Part print with two shaded views. Sizes in mm from the minimum x, y, z corner. A direction names the side the tool comes from. Coordinates: 2 decimals unless noted, no trailing zeros. Loops run counter-clockwise (first coordinate to the right, second up) from the corner with the lowest first, then second, coordinate; pieces in that order, holes last. Notation, with made-up numbers: (26.25, 20.25) -> (32.25, 20.25) arc R6 cw to (32.25, 27.25) -> close; hole circle Ø9 at (-34, -30.75). An arc over 180 degrees is marked (long way). Return JSON: item names as keys, results as strings. Group by question number.
(1) Saw through at C-C on y = 53.5. Write the cut outline in (x, z).
(2) Mould opens along Y. For the marked faces 3, 4, 5 and 6 say: pulls with the +Y half, pulls with the -Y half, needs draft (parallel to the pull), parting line crosses it, or undercut.
(3) Flat gauge pin, fed straight in: pin 1 Ø11 at (x, y) = (90, 22) entering from +Z. Where does the tip first touch, or does it go through?
(4) Saw through at D-D on z = 6.5. Write the cut outline in (x, y).
(5) Saw through at A-A on x = 39.5. Write the cut outline in (y, z), then the cut area to 3 significant figures.
(6) Probe L1, parallel to Y at x = 106.5, z = 1.55; L2, parallel to X at y = 84, z = 13; L3, parallel to Y at x = 114, z = 11. List the from-to ranges inside material, lowest first.
(7) Tool access for the marked faces 1 and 2: list every direction of +Z, -Z, +X, -X, +Y, -Y with a clear straight run to the whole face (end or side of a thin tool).
(8) Saw through at B-B on y = 87.5. Write the cut outline in (x, z), then the cut area to 3 significant figures.
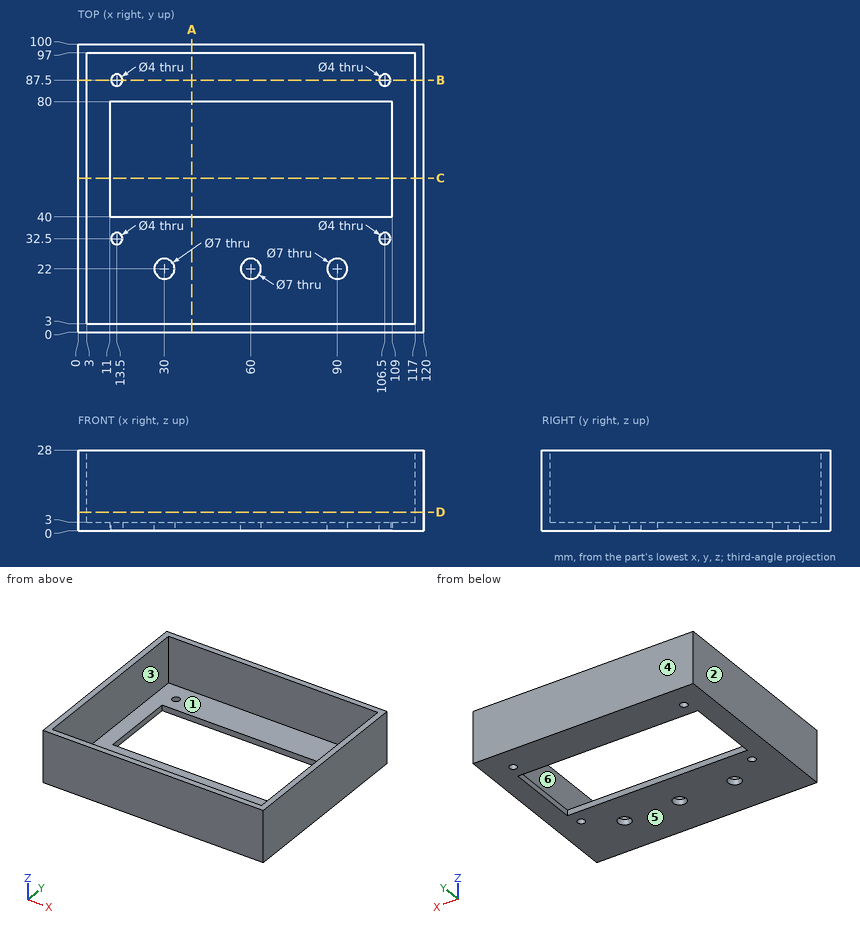
Geometry results:
{
 "1": {"outline": "(0, 0) -> (11, 0) -> (11, 3) -> (3, 3) -> (3, 28) -> (0, 28) -> close; (109, 0) -> (120, 0) -> (120, 28) -> (117, 28) -> (117, 3) -> (109, 3) -> close"},
 "2": {"face 3": "undercut", "face 4": "pulls with the +Y half", "face 5": "needs draft", "face 6": "undercut"},
 "3": {"pin 1": "z = 3"},
 "4": {"outline": "(0, 0) -> (120, 0) -> (120, 100) -> (0, 100) -> close; hole (3, 3) -> (117, 3) -> (117, 97) -> (3, 97) -> close"},
 "5": {"outline": "(0, 0) -> (40, 0) -> (40, 3) -> (3, 3) -> (3, 28) -> (0, 28) -> close; (80, 0) -> (100, 0) -> (100, 28) -> (97, 28) -> (97, 3) -> (80, 3) -> close", "area": "330 mm²"},
 "6": {"L1": "0 to 30.5, 34.5 to 40, 80 to 85.5, 89.5 to 100", "L2": "0 to 3, 117 to 120", "L3": "0 to 3, 97 to 100"},
 "7": {"face 1": "+Z", "face 2": "+Z, -Z, -X, +Y, -Y"},
 "8": {"outline": "(0, 0) -> (11.5, 0) -> (11.5, 3) -> (3, 3) -> (3, 28) -> (0, 28) -> close; (15.5, 0) -> (104.5, 0) -> (104.5, 3) -> (15.5, 3) -> close; (108.5, 0) -> (120, 0) -> (120, 28) -> (117, 28) -> (117, 3) -> (108.5, 3) -> close", "area": "486 mm²"}
}
